Geometry check sheet. Reference: the model listing, model coordinates, mm. Coordinates: 2 decimals unless noted, no trailing zeros. Write each loop counter-clockwise with the first axis right and the second up, starting at its lowest first coordinate (ties: lowest second). Pieces come first, ordered by that corner, then holes.
from build123d import *

# Parameters (mm, degrees)
CUT_EXTRUDE1_DEPTH = 1.0922
CUT_EXTRUDE2_DEPTH = 7.35


with BuildPart() as part:
    # Sketch1 → Revolve1 (revolve)
    with BuildSketch(Plane.XY):
        Polygon((-9.232559292, 19.989816719), (-5.422559292, 19.989816719), (-7.149759292, 18.643616719), (-7.149759292, 14.411514199), (-7.797290363, 13.639816719), (-9.232559292, 13.639816719), align=None)
    revolve(axis=Axis((-9.232559292, 19.989816719, 0), (0, -1, 0)))

    # Sketch2 → Cut-Extrude1 (cut)
    with BuildSketch(Plane(origin=(0, 19.989816719, 0), x_dir=(1, 0, 0), z_dir=(0, 1, 0))):
        Polygon((-9.926643575, 1.1938), (-8.548145113, 1.1938), (-7.851656024, 0.004194621), (-8.540905254, -1.189620065), (-9.919378278, -1.197994621), (-10.608627508, -0.004179935), align=None)
    extrude(amount=-CUT_EXTRUDE1_DEPTH, mode=Mode.SUBTRACT)

    # Sketch4 → Cut-Extrude2 (cut, through all)
    with BuildSketch(Plane(origin=(0, 19.989816719, 0), x_dir=(1, 0, 0), z_dir=(0, 1, 0))):
        Polygon((-13.85844337, 0), (-4.15558518, 0), (-6.419880254, 3.714859107), (-9.922461698, 4.192483849), (-13.787684149, 2.78614433), align=None)
    extrude(amount=-CUT_EXTRUDE2_DEPTH, mode=Mode.SUBTRACT)

    # Sketch5 → Cut-Revolve1 (revolve, cut)
    with BuildSketch(Plane(origin=(0, 0, 0), x_dir=(-1, 0, 0), z_dir=(0, 0, -1))):
        with BuildLine():
            Line((9.230162876, 18.529316719), (9.598462876, 18.529316719))
            Line((9.598462876, 18.529316719), (10.39700559, 18.897616719))
            Line((10.39700559, 18.897616719), (10.39700559, 19.741247113))
            ThreePointArc((10.39700559, 19.741247113), (10.546973564, 19.827359633), (10.606247963, 19.989816719))
            Line((10.606247963, 19.989816719), (10.353982568, 19.989816719))
            Line((10.353982568, 19.989816719), (9.230162876, 19.989816719))
            Line((9.230162876, 19.989816719), (9.230162876, 18.529316719))
        make_face()
    revolve(axis=Axis((-9.230162876, 18.897616719, 0), (0, 1, 0)), mode=Mode.SUBTRACT)

    # Mirror1: part across plane


with BuildPart() as part_1:
    add(part.part)
    add(part.part.mirror(Plane(origin=(-13.85844337, 13.639816719, 0), x_dir=(1, 0, 0), z_dir=(0, 0, 1))))


solid = part_1.part
1. Thickness scan on line 1 along Z through (x, y) = (-8.75, 19); line 2 along X through (y, z) = (15.75, -1); line 3 along X through (y, z) = (15.25, -0.75). Record the ranges inside material, lowest first.
Computed values:
line 1: z = -2.49 to -1.19, 1.19 to 2.49
line 2: x = -11.06 to -7.41
line 3: x = -11.18 to -7.29
2. Gauge pin test, flat ends, axial feed: pin 1 Ø2 at (x, z) = (-8.5, -2.5) entering from -Y; pin 2 Ø1 at (x, z) = (-7, 1.5) entering from -Y; pin 3 Ø1.3 at (x, z) = (-9, 0.5) entering from +Y. Record the tip position at first contact, or that the pin passes through.
Computed values:
pin 1: stops at y = 13.84
pin 2: stops at y = 18.73
pin 3: stops at y = 18.9
3. Sectioned sample at A-A, the plane y = 18.25. Record the boundary of the cut face in (x, z).
Computed values:
outline: circle Ø4.17 at (-9.23, 0)
4. Draft check along X on faces 1 (the flat face through (-11, 19.99, 0)), 2 (the flat face through (-8.2, 19.3, 0.6)). Enter one of: released by +X, released by -X, zero draft, split by the parting line, or undercut.
Computed values:
face 1: zero draft
face 2: undercut
